Autodesk Inventor part; units mm, degrees
ref_plane "YZ Plane" through (0, 0, 0) normal (1, 0, 0) x (0, 1, 0)
ref_plane "XZ Plane" through (0, 0, 0) normal (0, 1, 0) x (-1, 0, 0)
ref_plane "XY Plane" through (0, 0, 0) normal (0, 0, 1) x (1, 0, 0)
sketch "Sketch1" plane through (0, 0, 0) normal (0, 0, 1) x (1, 0, 0)
  circle A0 centre (0, 0) radius 32.25
  circle A1 centre (0, 0) radius 34
  line L0 (0, 0) -> (34, 0) construction
  line L1 (0, 0) -> (30.0202, 15.962) construction
  circle A2 centre (0, 0) radius 30.7
  line L2 (0, 0) -> (26.7199, 15.1174) construction
  line L3 (0, 0) -> (27.4745, 13.6983) construction
  line L4 (28.069, 15.8807) -> (29.5921, 16.7424) construction
  line L5 (28.8616, 14.3899) -> (30.4278, 15.1707) construction
  line L6 (27.4745, 13.6983) -> (28.8616, 14.3899)
  line L7 (26.7199, 15.1174) -> (28.069, 15.8807)
  line L8 (-26.7199, -15.1174) -> (-28.069, -15.8807)
  line L9 (-27.4745, -13.6983) -> (-28.8616, -14.3899)
  point P0 (-28.069, -15.8807)
  point P1 (-27.4745, -13.6983)
  dimension "d0" = 64.5
  dimension "d1" = 68
  dimension "d2" = 28
  dimension "d3" = 61.4
  dimension "d4" = 3
  dimension "d11" = 360
extrude "Extrusion1" add sketch "Sketch1" along normal blind 1.5 contours L6 A2 L7 A0 | A0 L9 A2 L8 | A1
sketch "Sketch2" plane through (0, 0, 0) normal (0, 0, -1) x (-1, 0, 0)
  line L0 (-27.4745, 13.6983) -> (-28.8616, 14.3899)
  arc A0 (-28.8616, 14.3899) -> (28.069, -15.8807) centre (0, 0) ccw
  line L1 (28.069, -15.8807) -> (26.7199, -15.1174)
  arc A1 (26.7199, -15.1174) -> (27.4745, -13.6983) centre (0, 0) ccw
  line L2 (27.4745, -13.6983) -> (28.8616, -14.3899)
  arc A2 (28.8616, -14.3899) -> (-28.069, 15.8807) centre (0, 0) ccw
  line L3 (-28.069, 15.8807) -> (-26.7199, 15.1174)
  arc A3 (-26.7199, 15.1174) -> (-27.4745, 13.6983) centre (0, 0) ccw
  circle A4 centre (0, 0) radius 34
  line L4 (0, 0) -> (-34, 0) construction
  arc A5 (-30.7, 0) -> (-29.8518, -7.1668) centre (0, 0) ccw
  arc A6 (-28.9137, -12.8732) -> (-30.0144, -10.0427) centre (0, 0) ccw construction
  line L5 (0, 0) -> (-28.0458, -12.4868) construction
  line L6 (-28.0458, -12.4868) -> (-28.5026, -12.6902) construction
  line L7 (0, 0) -> (-30.0144, -10.0427) construction
  line L8 (0, 0) -> (-30.7755, -7.3885) construction
  line L9 (-30.0144, -10.0427) -> (-29.8518, -7.1668)
  arc A7 (-23.1861, -20.8769) -> (-28.5026, -12.6902) centre (0, 0) ccw construction
  line L10 (0, 0) -> (-23.9664, -21.5795) construction
  line L11 (-28.5026, -12.6902) -> (-28.9137, -12.8732)
  line L12 (0, 0) -> (-19.8551, -25.4133) construction
  line L13 (-23.1861, -20.8769) -> (-19.8551, -25.4133)
  arc A8 (-30.0144, -10.0427) -> (-28.9137, -12.8732) centre (0, 0) ccw
  arc A9 (-28.5026, -12.6902) -> (-23.1861, -20.8769) centre (0, 0) ccw
  arc A10 (-27.4745, 13.6983) -> (-30.7, 0) centre (0, 0) ccw
  arc A11 (-29.8518, -7.1668) -> (-26.7199, 15.1174) centre (0, 0) ccw construction
  arc A12 (-26.7199, 15.1174) -> (-27.4745, 13.6983) centre (0, 0) ccw
  arc A13 (26.7199, -15.1174) -> (27.4745, -13.6983) centre (0, 0) ccw
  arc A14 (27.4745, -13.6983) -> (30.7, 0) centre (0, 0) ccw
  arc A15 (30.7, 0) -> (29.8518, 7.1668) centre (0, 0) ccw
  line L14 (30.0144, 10.0427) -> (29.8518, 7.1668)
  arc A16 (30.0144, 10.0427) -> (28.9137, 12.8732) centre (0, 0) ccw
  line L15 (28.5026, 12.6902) -> (28.9137, 12.8732)
  arc A17 (28.5026, 12.6902) -> (23.1861, 20.8769) centre (0, 0) ccw
  line L16 (23.1861, 20.8769) -> (19.8551, 25.4133)
  line L17 (0, 0) -> (6.3829, -30.0291) construction
  arc A18 (-28.8616, 14.3899) -> (28.069, -15.8807) centre (0, 0) ccw
  arc A19 (6.3829, -30.0291) -> (26.7199, -15.1174) centre (0, 0) ccw
  line L18 (6.3829, -30.0291) -> (6.7052, -31.5453)
  line L19 (0, 0) -> (-6.3829, 30.0291) construction
  line L20 (-6.3829, 30.0291) -> (-6.7052, 31.5453)
  arc A20 (-6.3829, 30.0291) -> (-26.7199, 15.1174) centre (0, 0) ccw
  point P0 (28.0458, 12.4868)
  point P1 (27.4745, -13.6983)
  point P2 (-26.7199, 15.1174)
  dimension "d15" = 63.3
  dimension "d16" = 24
  dimension "d17" = 18.5
  dimension "d18" = 13.5
  dimension "d19" = 62.4
  dimension "d20" = 42
  dimension "d21" = 52
  dimension "d24" = 360
  dimension "d43" = 50
  dimension "d46" = 360
extrude "Extrusion2" add sketch "Sketch2" along normal blind 1.65 contours A10 A5 L9 A8 L11 A9 L13 A0 L0 | L3 A2 L20 A20 | L18 A19 L1 A0 | A2 L2 A14 A15 L14 A16 L15 A17 L16 | A4
sketch "Sketch4" plane through (0, 0, 1.5) normal (0, 0, 1) x (1, 0, 0)
  circle A0 centre (0, 0) radius 34
  arc A1 (28.069, 15.8807) -> (-28.8616, -14.3899) centre (0, 0) ccw
  circle A2 centre (0, 0) radius 32.25
  point P0 (-28.8616, -14.3899)
extrude "Extrusion4" add sketch "Sketch4" along normal blind 56.6
sketch "Sketch5" plane through (0, 0, 58.1) normal (0, 0, 1) x (1, 0, 0)
  circle A0 centre (0, 0) radius 34
  line L0 (-20, 13) -> (20, 13)
  line L1 (20, 13) -> (20, -13)
  line L2 (20, -13) -> (-20, -13)
  line L3 (-20, -13) -> (-20, 13)
  line L4 (-20, 13) -> (20, -13) construction
  line L5 (20, 13) -> (-20, -13) construction
  dimension "d37" = 40
  dimension "d38" = 26
extrude "Extrusion5" add sketch "Sketch5" against normal blind 2
sketch "Sketch6" plane through (0, 0, 56.1) normal (0, 0, -1) x (-1, 0, 0)
  line L0 (-20, 13) -> (20, 13)
  line L1 (20, 13) -> (20, -13)
  line L2 (20, -13) -> (-20, -13)
  line L3 (-20, -13) -> (-20, 13)
  circle A0 centre (0, 0) radius 32.25
  line L4 (-20, -13) -> (20, -13)
  line L5 (20, -13) -> (20, -25.2995)
  line L6 (20, -13) -> (20, 13) construction
  line L7 (20, 0) -> (-20, 0) construction
  line L8 (-20, 13) -> (-20, -13) construction
  line L9 (0, -13) -> (0, 13) construction
  line L10 (20, 13) -> (-20, 13) construction
  line L11 (-20, -13) -> (-20, -25.2995)
  line L12 (20, 13) -> (20, 25.2995)
  line L13 (-20, 13) -> (-20, 25.2995)
extrude "Extrusion6" add sketch "Sketch6" along normal blind 0.6 contours L3 L11 A0 L13 | L12 A0 L5 L1
properties part number "LensMount"
The model under review builds one solid part; all positions refer to its coordinate system, in mm. A direction names the side the tool comes from. Round coordinates to 2 decimals unless told otherwise and drop trailing zeros. Write each loop counter-clockwise with the first axis right and the second up, starting at its lowest first coordinate (ties: lowest second). Pieces come first, ordered by that corner, then holes.
(1) Insertion check: pin 1 (12 mm diameter, centred on x = 18.5, z = 20.5, fed in from -Y); pin 2 (1 mm diameter, centred on y = 9, z = 36, fed in from -X); pin 3 (1.3 mm diameter, centred on y = -9, z = 57.5, fed in from -X). Each pin has a flat end and moves straight along its axis. Give the tip position at first contact, or say it passes through.
(2) We need section C-C on z = 29.5. Give the boundary of the cut face in (x, y).
(3) We need section A-A on x = 0. Give the boundary of the cut face in (y, z), and give its area (3 significant figures).
(4) Wall thickness on L1, parallel to X at y = 0.5, z = 47.5; L2, parallel to Y at x = 1, z = 45; L3, parallel to Z at x = 3, y = -30: over which ranges is each line inside the solid? List them lowest first.
(5) We need section B-B on y = -11. Give the boundary of the cut face in (x, z).
(6) We need section D-D on y = 17. Give the boundary of the cut face in (x, z).
(7) Mouldability with a two-part tool opening along X and no side actions: class faces 1 (the flat face through (-25, 0, 55.5)), 2 (the flat face through (-7.4, -30.1, -1.65)) as +X half, -X half, draft (parallel to the pull), parting line (faces both ways), or undercut.
(8) Machinability: for faces 3 (the flat face through (18.1, 25.2, 0)), 4 (the flat face through (0, 13, 57)), 5 (the flat face through (21.544, -23.113, -0.813)), which of the approach directions +Z, -Z, +X, -X, +Y, -Y give a long, thin tool a straight path to every point of the face, cutting with its end or side? Answer none if there is none.
Findings below:
1. pin 1: stops at y = -31.62
1. pin 2: stops at x = -32.92
1. pin 3: stops at x = -32.96
2. outline: circle Ø68 at (0, 0); hole (-28.86, -14.39) arc R32.25 ccw (long way) to (28.07, 15.88) arc R32.25 ccw to start
3. outline: (-34, -1.65) - (-32.25, -1.65) - (-32.25, 56.1) - (-13, 56.1) - (-13, 58.1) - (-34, 58.1) - close; (13, 56.1) - (32.25, 56.1) - (32.25, 0) - (32.25, -1.65) - (34, -1.65) - (34, 58.1) - (13, 58.1) - close
3. area: 286 mm2
4. L1: x = -34 to -32.25, 32.25 to 34
4. L2: y = -33.99 to -32.23, 32.23 to 33.99
4. L3: z = 56.1 to 58.1
5. outline: (-32.17, -1.65) - (-28.66, -1.65) - (-28.66, 0) - (-30.32, 0) - (-30.32, 55.5) - (-20, 55.5) - (-20, 58.1) - (-32.17, 58.1) - close; (20, 55.5) - (30.32, 55.5) - (30.32, 0) - (29.68, 0) - (29.68, -1.65) - (32.17, -1.65) - (32.17, 58.1) - (20, 58.1) - close
6. outline: (-29.44, -1.65) - (-26.16, -1.65) - (-26.16, 0) - (-27.41, 0) - (-27.41, 55.5) - (-20, 55.5) - (-20, 56.1) - (20, 56.1) - (20, 55.5) - (27.41, 55.5) - (27.41, 0) - (25.56, 0) - (25.56, -1.65) - (29.44, -1.65) - (29.44, 58.1) - (-29.44, 58.1) - close
7. face 1: undercut
7. face 2: draft
8. face 3: none
8. face 4: +Z, -Z
8. face 5: -Z
